Design review of the part built by this model. Coordinates are the model's own, in mm. Round coordinates to 2 decimals unless told otherwise and drop trailing zeros. Loops run counter-clockwise (first coordinate to the right, second up) from the corner with the lowest first, then second, coordinate; pieces in that order, holes last. Notation, with made-up numbers: (26.25, 39.5) -> (39.25, 39.5) arc R12 ccw to (39.25, 49.5) -> close; hole circle Ø8 at (49.5, 59). An arc over 180 degrees is marked (long way). Use a Markdown table: item, result. Add a question column.
from build123d import *

# Parameters (mm, degrees)
F0_R     = 18
F0_R_2   = 10.5
F1_DEPTH = 4
F2_SIZE  = 2


# Not quite as in the source:
# - a feature names something its author has since deleted; it is built from what else it names


with BuildPart() as f1:
    # F0 (on Top) → F1 (new body)
    with BuildSketch(Plane.XY):
        with BuildLine():
            ThreePointArc((-55.5, 32.5), (-87.5, 0), (-55.5, -32.5))
            Line((-55.5, -32.5), (55.5, -32.5))
            ThreePointArc((55.5, -32.5), (87.5, 0), (55.5, 32.5))
            Line((55.5, 32.5), (-55.5, 32.5))
        make_face()
        with Locations((-55, 0)):
            Circle(F0_R, mode=Mode.SUBTRACT)
        with Locations((60, 0)):
            Circle(F0_R_2, mode=Mode.SUBTRACT)
    extrude(amount=F1_DEPTH)

    # F2
    f2_edges = [f1.edges().sort_by_distance(p)[0] for p in [
        (-73, 0, 4),
        (49.5, 0, 4),
    ]]
    chamfer(f2_edges, length=F2_SIZE)


solid = f1.part
1. Mouldability with a two-part tool opening along Y and no side actions: class faces 1 (the face through (1, 32.5, 2)), 2 (the face through (-1, -32.5, 2)), 3 (the face through (-37.712, 5.444, 2.125)) as +Y half, -Y half, draft (parallel to the pull), parting line (faces both ways), or undercut.
2. Consider section D-D on y = 25. State the section outline as (x, z) points, plus the area to 3 significant figures.
3. To check wall thickness, follow probe 1 along Y at (x, z) = (-55, 0.4); probe 2 along X at (y, z) = (3.5, 3.8); probe 3 along X at (y, z) = (-4, 2.45). State the ranges of each line that lie inside material, in increasing order. Write a range as from..to.
4. Consider section B-B on x = 60. State the section outline as (y, z) points.
5. Consider section C-C on y = -3. Give the number of separate pieces and of enclosed holes in the cut face, plus the area to 3 significant figures.
Verdict:
| question | item | result |
|---|---|---|
| 1 | face 1 | +Y half |
| 1 | face 2 | -Y half |
| 1 | face 3 | undercut |
| 2 | outline | (-75.77, 0) -> (75.77, 0) -> (75.77, 4) -> (-75.77, 4) -> close |
| 2 | area | 606 mm² |
| 3 | probe 1 | y = -32.5..-18, 18..32.5 |
| 3 | probe 2 | x = -87.31..-74.49, -35.51..48.21, 71.79..87.31 |
| 3 | probe 3 | x = -87.25..-73.01, -36.99..49.81, 70.19..87.25 |
| 4 | outline | (-32.12, 0) -> (-10.5, 0) -> (-10.5, 2) -> (-12.5, 4) -> (-32.12, 4) -> close; (10.5, 0) -> (32.12, 0) -> (32.12, 4) -> (12.5, 4) -> (10.5, 2) -> close |
| 5 | separate pieces | 3 |
| 5 | enclosed holes | 0 |
| 5 | area | 468 mm² |
